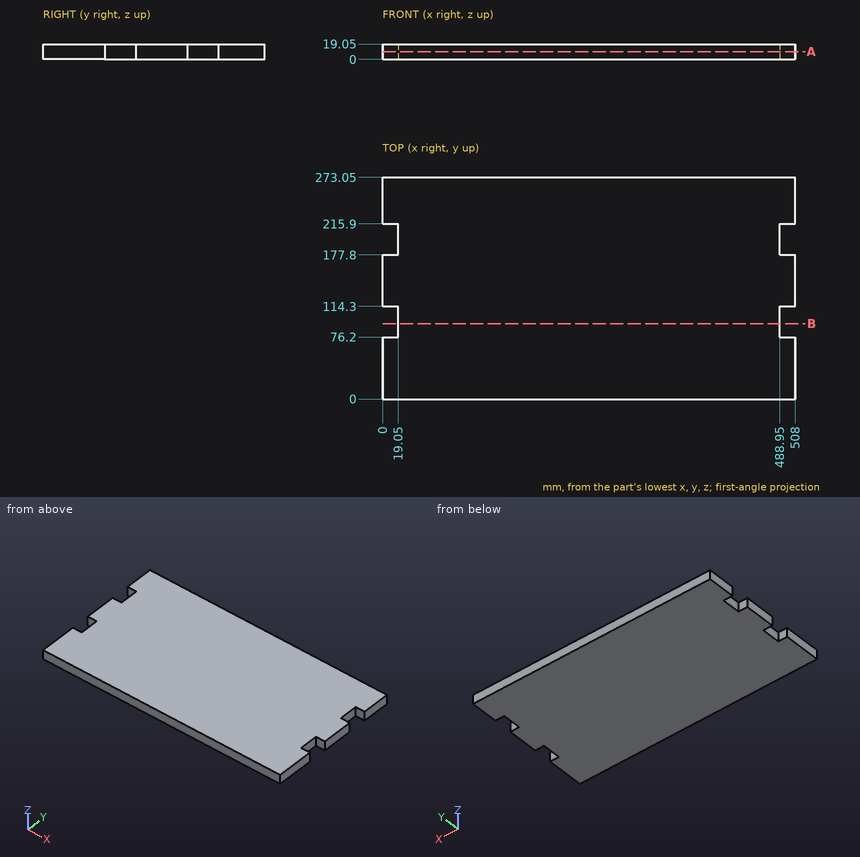
Can you work these out from the drawing? Everything is in mm from the part's minimum corner. Coordinates: 2 decimals unless noted, no trailing zeros. Loops run counter-clockwise (first coordinate to the right, second up) from the corner with the lowest first, then second, coordinate; pieces in that order, holes last. Notation, with made-up numbers: M 5.5,84.25 L 27.5,84.25 A13 cw 27.5,97.25 Z; hole C 35.5,-10.5 d8. An arc over 180 degrees is marked long. Put each result on its own line as item: value. Start each with the question number.
(1) Will these pins go through, and if not, where does the flat tip stop? P1, Ø9.5, axis at y = 204, z = 13.5, coming from the -X side; P2, Ø9.5, axis at y = 203, z = 8, coming from the +X side.
(2) I need wall thicknesses on line 1 (X direction, y = 208, z = 2). Which ranges of the line are inside material? Lowest first, please. Write a range as from..to.
(3) Suppose I cut it at B-B on y = 93. Please give me the cut outline in (x, z).
(4) Suppose I cut it at A-A on z = 9.5. Please give me the cut outline in (x, y).
Solutions:
1. P1: stops at x = 19.05
1. P2: stops at x = 488.95
2. line 1: x = 19.05..488.95
3. outline: M 19.05,0 L 488.95,0 L 488.95,19.05 L 19.05,19.05 Z
4. outline: M 0,0 L 508,0 L 508,76.2 L 488.95,76.2 L 488.95,114.3 L 508,114.3 L 508,177.8 L 488.95,177.8 L 488.95,215.9 L 508,215.9 L 508,273.05 L 0,273.05 L 0,215.9 L 19.05,215.9 L 19.05,177.8 L 0,177.8 L 0,114.3 L 19.05,114.3 L 19.05,76.2 L 0,76.2 Z
